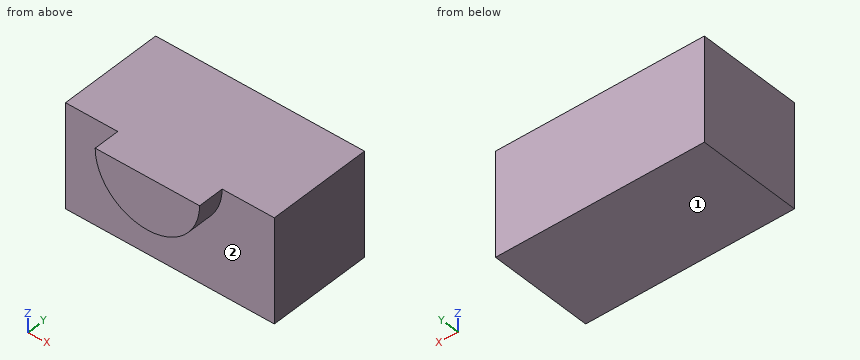
from build123d import *

# Parameters (mm, degrees)
F0_W     = 2032
F0_H     = 1016
F1_DEPTH = 1016
F3_DEPTH = 254
F5_DEPTH = 1016


with BuildPart() as f1:
    # F0 (on Top) → F1 (new body)
    with BuildSketch(Plane.XY):
        with Locations((-455.675927, 199.958904)):
            Rectangle(F0_W, F0_H)
    extrude(amount=F1_DEPTH)

    # F2 (on face) → F3 (join)
    with BuildSketch(Plane.XZ.offset(308.041096)):
        with BuildLine():
            Line((-709.675927, 1016), (-963.675927, 1016))
            ThreePointArc((-963.675927, 1016), (-455.675927, 508.736016), (52.324073, 1016))
            Line((52.324073, 1016), (-201.675927, 1016))
            ThreePointArc((-201.675927, 1016), (-455.675927, 763.618704), (-709.675927, 1016))
        make_face()
        with BuildLine():
            Line((-201.675927, 1016), (-709.675927, 1016))
            ThreePointArc((-709.675927, 1016), (-455.675927, 763.618704), (-201.675927, 1016))
        make_face()
    extrude(amount=F3_DEPTH)

    # F4 (on face) → F5 (join)
    with BuildSketch(Plane.XZ.offset(562.041096)):
        with BuildLine():
            Line((-201.675927, 1016), (-709.675927, 1016))
            ThreePointArc((-709.675927, 1016), (-455.675927, 763.326984), (-201.675927, 1016))
        make_face()
    extrude(amount=-F5_DEPTH)


solid = f1.part
Input: part model. Units: mm. Frame: model coordinates. Face numbers are marked on the shaded views. A direction names the side the tool comes from. Round coordinates to 2 decimals unless told otherwise and drop trailing zeros. Write each loop counter-clockwise with the first axis right and the second up, starting at its lowest first coordinate (ties: lowest second). Pieces come first, ordered by that corner, then holes.
1) Ray query, L1, parallel to Y at x = -24, z = 329.5. Return the intervals inside material, ascending.
2) Cut plane B-B (x = -308). Return the cut outline in (y, z), then the cut area to 3 significant figures.
3) Cut plane D-D (x = -45.5). Return the cut outline in (y, z).
4) Cut plane C-C (z = 377.5). Return the cut outline in (x, y).
5) Cut plane A-A (y = -404). Return the cut outline in (x, z).
6) Reachability of the marked faces 1 and 2 from +Z, -Z, +X, -X, +Y, -Y: full face, straight path, thin tool, end or side. Return the list, or none.
Geometry says:
1. L1: y = -308.04 to 707.96
2. outline: (-562.04, 530.67) - (-308.04, 530.67) - (-308.04, 0) - (707.96, 0) - (707.96, 1016) - (-562.04, 1016) - close
2. area: 1,160,000 mm2
3. outline: (-562.04, 717.04) - (-308.04, 717.04) - (-308.04, 0) - (707.96, 0) - (707.96, 1016) - (-562.04, 1016) - close
4. outline: (-1471.68, -308.04) - (560.32, -308.04) - (560.32, 707.96) - (-1471.68, 707.96) - close
5. outline: (-963.68, 1016) arc R508 ccw to (52.32, 1016) - close
6. face 1: -Z, +X, -X, +Y, -Y
6. face 2: -Z, -Y
